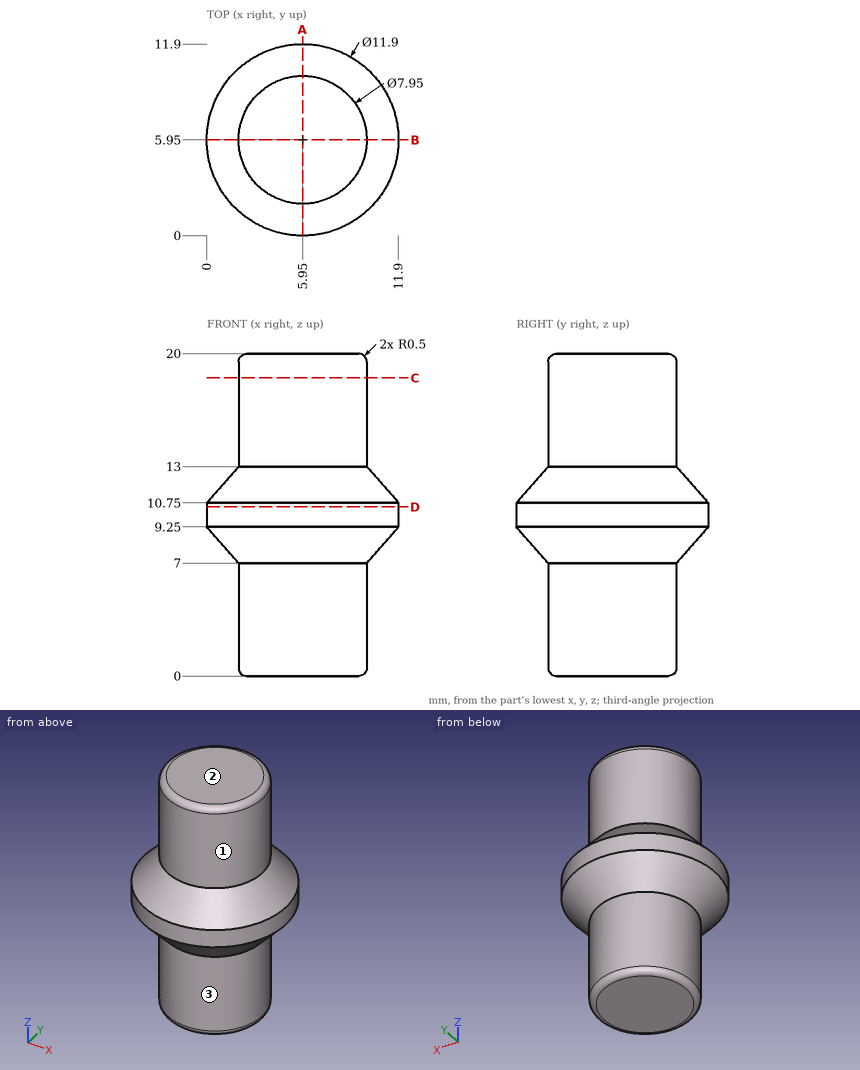
Input: dimensioned drawing with shaded views. Units: mm. Origin: part minimum x, y, z. A direction names the side the tool comes from. Round coordinates to 2 decimals unless told otherwise and drop trailing zeros. Loops run counter-clockwise (first coordinate to the right, second up) from the corner with the lowest first, then second, coordinate; pieces in that order, holes last. Notation, with made-up numbers: (26.5, 9.5) -> (55.5, 9.5) arc R12 ccw to (55.5, 17.5) -> close; hole circle Ø1 at (53, -5.75). An arc over 180 degrees is marked (long way). Use one line per item in the form item = value. Start each with the question number.
1) Section C-C on z = 18.5. Output: boundary loops of the cut face in (x, y) (3 decimals), then the cut area to 3 significant figures.
2) Access query for the marked faces 1, 2 and 3. Directions: +Z, -Z, +X, -X, +Y, -Y. A direction counts if a zero-diameter tool reaches every point of the face in a straight line with its end or side. Return the directions, or none.
3) Section A-A on x = 5.95. Output: boundary loops of the cut face in (y, z) (3 decimals).
4) Line query: L1, parallel to X at y = 7, z = 8; L2, parallel to Z at x = 4.5, y = 10.75; L3, parallel to Y at x = 2.75, z = 4. Output: solid intervals per line, ascending.
5) Section D-D on z = 10.5. Output: boundary loops of the cut face in (x, y).
6) First-contact query: P1, Ø4, axis at x = 1, z = 2, coming from the -Y side; P2, Ø3, axis at y = 3.5, z = 2, coming from the -X side; P3, Ø4, axis at y = 9, z = 13.5, coming from the +X side. Flat tips, straight axial feed; report the tip coordinate or a pass-through.
Response:
q1.outline = circle Ø7.95 at (5.95, 5.95)
q1.area = 49.6 mm^2
q2.face_1 = +Z
q2.face_2 = +Z, +X, -X, +Y, -Y
q2.face_3 = -Z
q3.outline = (0, 9.25) -> (1.975, 7) -> (1.975, 0.5) arc R0.5 ccw to (2.475, 0) -> (9.425, 0) arc R0.5 ccw to (9.925, 0.5) -> (9.925, 7) -> (11.9, 9.25) -> (11.9, 10.75) -> (9.925, 13) -> (9.925, 19.5) arc R0.5 ccw to (9.425, 20) -> (2.475, 20) arc R0.5 ccw to (1.975, 19.5) -> (1.975, 13) -> (0, 10.75) -> close
q4.L1 = 1.21 to 10.69
q4.L2 = 8.18 to 11.82
q4.L3 = 3.59 to 8.31
q5.outline = circle Ø11.9 at (5.95, 5.95)
q6.P1 = 3.29
q6.P2 = 2.09
q6.P3 = 10.58
